```python
from build123d import *

# Parameters (mm, degrees)
ESBO_O1_R                = 8.05
RESSALTO_EXTRUS_O1_DEPTH = 4
ESCALA1_SCALE            = 0.95
ESBO_O2_R                = 8.25
ESBO_O2_R_2              = 7.6475
CORTE_EXTRUS_O1_DEPTH    = 10


with BuildPart() as part:
    # Esboço1 → Ressalto-extrusão1 (new body)
    with BuildSketch(Plane.XY):
        with BuildLine():
            Line((-9.55, -16.1), (-11.2, -16.1))
            Line((-11.2, -16.1), (-11.2, -18.526258263))
            Line((-11.2, -18.526258263), (-11.2, -19.1))
            Line((-11.2, -19.1), (12.8, -19.1))
            Line((12.8, -19.1), (12.8, -18.526258263))
            Line((12.8, -18.526258263), (12.8, -16.1))
            Line((12.8, -16.1), (11.15, -16.1))
            Line((11.15, -16.1), (11.15, -12))
            Line((11.15, -12), (12.8, -12))
            Line((12.8, -12), (12.8, -9.47671964))
            Line((12.8, -9.47671964), (16, -9.47671964))
            Line((16, -9.47671964), (16, -12))
            Line((16, -12), (17.65, -12))
            Line((17.65, -12), (17.65, -16.1))
            Line((17.65, -16.1), (16, -16.1))
            Line((16, -16.1), (16, -18.526258263))
            Line((16, -18.526258263), (16, -19.1))
            Line((16, -19.1), (25.4, -19.1))
            Line((25.4, -19.1), (25.4, 2))
            ThreePointArc((25.4, 2), (22.471067812, 9.071067812), (15.4, 12))
            Line((15.4, 12), (-13.8, 12))
            ThreePointArc((-13.8, 12), (-20.871067812, 9.071067812), (-23.8, 2))
            Line((-23.8, 2), (-23.8, -19.1))
            Line((-23.8, -19.1), (-14.4, -19.1))
            Line((-14.4, -19.1), (-14.4, -16.1))
            Line((-14.4, -16.1), (-16.05, -16.1))
            Line((-16.05, -16.1), (-16.05, -12))
            Line((-16.05, -12), (-14.4, -12))
            Line((-14.4, -12), (-14.4, -9.47671964))
            Line((-14.4, -9.47671964), (-11.2, -9.47671964))
            Line((-11.2, -9.47671964), (-11.2, -12))
            Line((-11.2, -12), (-9.55, -12))
            Line((-9.55, -12), (-9.55, -16.1))
        make_face()
        with Locations((-12.8, 1)):
            Circle(ESBO_O1_R, mode=Mode.SUBTRACT)
        with Locations((14.4, 1)):
            Circle(ESBO_O1_R, mode=Mode.SUBTRACT)
    extrude(amount=RESSALTO_EXTRUS_O1_DEPTH)


with BuildPart() as part_1:
    # Escala1: scaled about (0.8, -5.041502423, 2)
    add(part.part.scale(ESCALA1_SCALE).moved(Location((0.04, -0.252075121, 0.1))))

    # Esboço2 → Corte-extrusão1 (cut)
    # profile 1 of 2: a face of its own
    with BuildSketch(Plane(origin=(0, 0, 0.1), x_dir=(-1, 0, 0), z_dir=(0, 0, -1))):
        with Locations((12.12, 0.697924879)):
            Circle(ESBO_O2_R)
        with Locations((12.12, 0.697924879)):
            Circle(ESBO_O2_R_2, mode=Mode.SUBTRACT)
    # profile 2 of 2: a face of its own
    with BuildSketch(Plane(origin=(0, 0, 0.1), x_dir=(-1, 0, 0), z_dir=(0, 0, -1))):
        with Locations((-13.72, 0.697924879)):
            Circle(ESBO_O2_R)
        with Locations((-13.72, 0.697924879)):
            Circle(ESBO_O2_R_2, mode=Mode.SUBTRACT)
    extrude(amount=-CORTE_EXTRUS_O1_DEPTH, mode=Mode.SUBTRACT)


solid = part_1.part
```
Check sheet for the modelled part. Datum: model origin and axes. Units: mm. A direction names the side the tool comes from. Round coordinates to 2 decimals unless told otherwise and drop trailing zeros. Order: outer loops, then holes, each group sorted by start corner. A loop starts at its lowest first (then second) coordinate and runs counter-clockwise, first axis right, second up. Notation, with made-up numbers: M -1.5,-38.75 L 53.5,-38.75 A14 ccw 53.5,-26.75 Z; hole C -8,18 d10. An arc over 180 degrees is marked long. Answer in a Markdown table with one row per item.
(1) Section check C-C on z = 2. Give the number of separate pieces and of enclosed holes in the cut face, plus the area to 3 significant figures.
Findings:
| item | result |
|---|---|
| separate pieces | 1 |
| enclosed holes | 2 |
| area | 835 mm^2 |
(2) Section check A-A on x = -12.12. Record the boundary of the cut face in (y, z).
Findings:
| item | result |
|---|---|
| outline | M -9.25,0.1 L -7.55,0.1 L -7.55,3.9 L -9.25,3.9 Z; M 8.95,0.1 L 11.15,0.1 L 11.15,3.9 L 8.95,3.9 Z |
(3) Gauge pin test, flat ends, axial feed: pin 1 (0.5 mm diameter, centred on x = 15.5, z = 2.5, fed in from +Y); pin 2 (8 mm diameter, centred on x = -10.5, y = 6, fed in from +Z); pin 3 (1.5 mm diameter, centred on x = -12, z = 2.5, fed in from -Y). Record the tip position at first contact, or that the pin passes through.
Findings:
| item | result |
|---|---|
| pin 1 | stops at y = 11.13 |
| pin 2 | stops at z = 3.9 |
| pin 3 | stops at y = -9.25 |
(4) Draft check along Y on faces 1 (the cylindrical face through (21.46, 8.29, 1.97)), 2 (the flat face through (-12, -9.255, 2)), 3 (the flat face through (0, -3, 3.9)), 4 (the cylindrical face through (-19.74, -2.46, 1.97)). Enter one of: +Y half, -Y half, draft (parallel to the pull), parting line (faces both ways), or undercut.
Findings:
| item | result |
|---|---|
| face 1 | +Y half |
| face 2 | -Y half |
| face 3 | draft |
| face 4 | undercut |
(5) Material ranges on line 1 along X through (y, z) = (-13.75, 3); line 2 along X through (y, z) = (2.5, 0.45); line 3 along Y through (x, z) = (-12.12, 2.2), recorded low to high. Write a range as from..to.
Findings:
| item | result |
|---|---|
| line 1 | x = -22.57..-15.21, -9.03..10.63, 16.81..24.17 |
| line 2 | x = -22.53..-20.17, -4.07..5.67, 21.77..24.13 |
| line 3 | y = -9.25..-7.55, 8.95..11.15 |
(6) Section check B-B on y = -13.25. Record the boundary of the cut face in (x, z), plus the area to 3 significant figures.
Findings:
| item | result |
|---|---|
| outline | M -22.57,0.1 L -15.21,0.1 L -15.21,3.9 L -22.57,3.9 Z; M -9.03,0.1 L 10.63,0.1 L 10.63,3.9 L -9.03,3.9 Z; M 16.81,0.1 L 24.17,0.1 L 24.17,3.9 L 16.81,3.9 Z |
| area | 131 mm^2 |
(7) Set-up check for faces 5 (the flat face through (11, -11.652, 2)), 6 (the flat face through (1, -18.397, 2)), 7 (the flat face through (-13.64, -10, 2)): record each of +Z, -Z, +X, -X, +Y, -Y from which the full face is reachable in a straight line by a thin tool's end or side.
Findings:
| item | result |
|---|---|
| face 5 | +Z, -Z |
| face 6 | +Z, -Z, +X, -X, -Y |
| face 7 | +Z, -Z, -Y |
(8) Section check D-D on x = -19. Record the boundary of the cut face in (y, z).
Findings:
| item | result |
|---|---|
| outline | M -18.4,0.1 L -3.85,0.1 L -3.85,3.9 L -18.4,3.9 Z; M 5.25,0.1 L 9.07,0.1 L 9.07,3.9 L 5.25,3.9 Z |
